Build history of the part. All positions in model axes, mm. Face numbers are marked on the shaded views. A direction names the side the tool comes from. Round coordinates to 2 decimals unless told otherwise and drop trailing zeros. Loops run counter-clockwise (first coordinate to the right, second up) from the corner with the lowest first, then second, coordinate; pieces in that order, holes last.
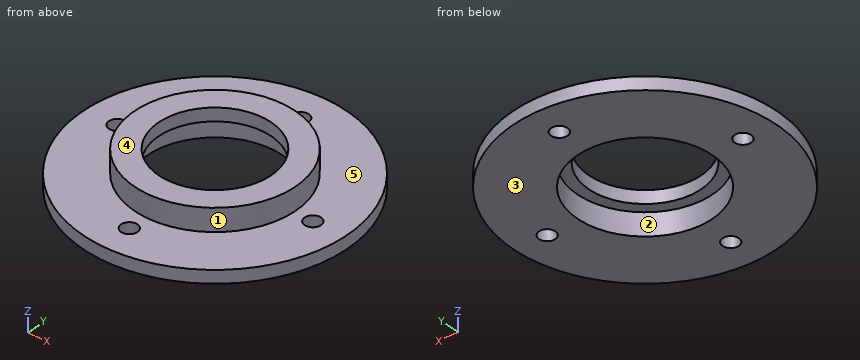
Autodesk Inventor part; units mm, degrees
ref_plane "YZ Plane" through (0, 0, 0) normal (1, 0, 0) x (0, 1, 0)
ref_plane "XZ Plane" through (0, 0, 0) normal (0, 1, 0) x (-1, 0, 0)
ref_plane "XY Plane" through (0, 0, 0) normal (0, 0, 1) x (1, 0, 0)
sketch "Sketch1" plane through (0, 0, 0) normal (0, 0, 1) x (1, 0, 0)
  circle A0 centre (0, 0) radius 21
  circle A1 centre (0, 0) radius 41
  circle A2 centre (0, 0) radius 31 construction
  circle A3 centre (0, 31) radius 2.55
  circle A4 centre (-31, 0) radius 2.55
  circle A5 centre (0, -31) radius 2.55
  circle A6 centre (31, 0) radius 2.55
  dimension "d0" = 42
  dimension "d1" = 20
  dimension "d2" = 10
  dimension "d3" = 5.1
  dimension "d6" = 360
extrude "Extrusion1" add sketch "Sketch1" along normal blind 4
sketch "Sketch2" plane through (0, 0, 4) normal (0, 0, 1) x (1, 0, 0)
  circle A0 centre (0, 0) radius 25
  circle A1 centre (0, 0) radius 21
  dimension "d10" = 4
extrude "Extrusion2" add sketch "Sketch2" along normal blind 3
sketch "Sketch3" plane through (0, 0, 7) normal (0, 0, 1) x (1, 0, 0)
  circle A0 centre (0, 0) radius 25
  circle A1 centre (0, 0) radius 17.5
  dimension "d13" = 35
extrude "Extrusion3" add sketch "Sketch3" along normal blind 4
properties part number "BearingHolder"
(1) Which spindle directions (+Z, -Z, +X, -X, +Y, -Y) get a long thin tool onto all of the face, cutting with end or side? Do the marked faces 4 and 5. Say none if no direction does.
Responses:
face 4: +Z, +X, -X, +Y, -Y
face 5: +Z
(2) Slice it at C-C on x = 31. List the corners of the cut face in (y, z), plus the area to 3 significant figures.
Responses:
outline: (-26.83, 0) - (-2.55, 0) - (-2.55, 4) - (-26.83, 4) - close; (2.55, 0) - (26.83, 0) - (26.83, 4) - (2.55, 4) - close
area: 194 mm2
(3) Slice it at D-D on z = 3. List the corners of the cut face in (x, y).
Responses:
outline: circle Ø82 at (0, 0); hole circle Ø5.1 at (-31, 0); hole circle Ø42 at (0, 0); hole circle Ø5.1 at (0, -31); hole circle Ø5.1 at (0, 31); hole circle Ø5.1 at (31, 0)
(4) Pull direction X, two halves, no side cores. Call the marked faces 1, 2 and 3: +X half, -X half, draft (parallel to the pull), parting line (faces both ways), or undercut.
Responses:
face 1: parting line
face 2: undercut
face 3: draft
(5) Pin check, flat tips, straight feed: P1, Ø5, axis at y = 9, z = 1.5, coming from the +X side; P2, Ø5, axis at y = -13, z = 3, coming from the +X side; P3, Ø6, axis at x = 0, y = 31, coming from the +Z side. Stop position of each tip, or through.
Responses:
P1: stops at x = 40.48
P2: stops at x = 39.63
P3: stops at z = 4
(6) Probe line 1 (Y direction, x = 0, z = 1); line 2 (Y direction, x = 0, z = 9.2); line 3 (Z direction, x = -2, y = -27). List the from-to ranges inside material, lowest first.
Responses:
line 1: y = -41 to -33.55, -28.45 to -21, 21 to 28.45, 33.55 to 41
line 2: y = -25 to -17.5, 17.5 to 25
line 3: z = 0 to 4
(7) Slice it at A-A on x = 0. List the corners of the cut face in (y, z), plus the area to 3 significant figures.
Responses:
outline: (-41, 0) - (-33.55, 0) - (-33.55, 4) - (-41, 4) - close; (-28.45, 0) - (-21, 0) - (-21, 7) - (-17.5, 7) - (-17.5, 11) - (-25, 11) - (-25, 4) - (-28.45, 4) - close; (17.5, 7) - (21, 7) - (21, 0) - (28.45, 0) - (28.45, 4) - (25, 4) - (25, 11) - (17.5, 11) - close; (33.55, 0) - (41, 0) - (41, 4) - (33.55, 4) - close
area: 203 mm2
(8) Slice it at B-B on y = -8.5. List the corners of the cut face in (x, z).
Responses:
outline: (-40.11, 0) - (-19.2, 0) - (-19.2, 7) - (-15.3, 7) - (-15.3, 11) - (-23.51, 11) - (-23.51, 4) - (-40.11, 4) - close; (15.3, 7) - (19.2, 7) - (19.2, 0) - (40.11, 0) - (40.11, 4) - (23.51, 4) - (23.51, 11) - (15.3, 11) - close
